Source: CAD feature listing. Evaluate the final solid. Frame: model axes, mm. Give positions to 0.01 mm unless a question says otherwise; leave off trailing zeros. Order: outer loops, then holes, each group sorted by start corner. A loop starts at its lowest first (then second) coordinate and runs counter-clockwise, first axis right, second up. Notation, with made-up numbers: M 23.25,73 L 80.25,73 A20 cw 80.25,112 Z; hole C -2.5,34.5 d5. An arc over 180 degrees is marked long. Answer as a JSON object with one key per item and string values. Group by question number.
1. Material intervals for L1, parallel to Y at x = 37, z = 0.25; L2, parallel to Y at x = 68, z = 0.8; L3, parallel to X at y = 65, z = 1.2 (3 decimals), sorted ascending. Write a range as [from, to].
2. Section query C-C (x = 57.15). Output: boundary loops of the cut face in (y, z), plus the area to 3 significant figures.
3. Section query A-A (x = 38). Output: boundary loops of the cut face in (y, z).
4. Section query D-D (y = 57). Output: boundary loops of the cut face in (x, z) (3 decimals).
5. Section query B-B (y = 68.35). Output: boundary loops of the cut face in (x, z) (3 decimals), plus the area to 3 significant figures.
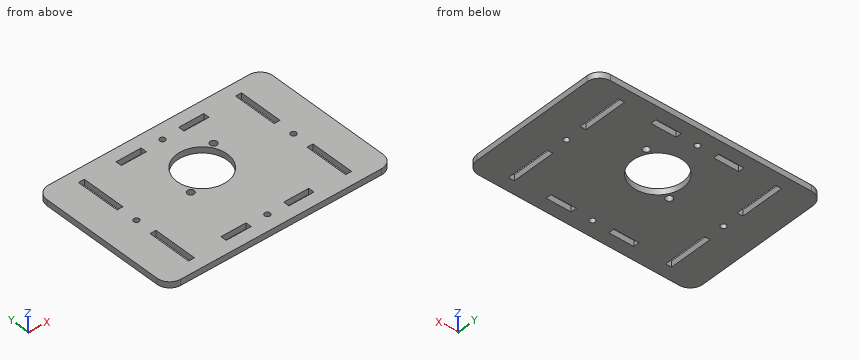
from build123d import *

# Parameters (mm, degrees)
BOSS_EXTRUDE1_DEPTH = 3
CUT_EXTRUDE1_REACH  = 139.404
SKETCH2_W           = 12.7
SKETCH2_H           = 3
SKETCH2_W_2         = 3
SKETCH2_H_2         = 22.225
CUT_EXTRUDE3_REACH  = 139.404
SKETCH4_R           = 1.7272
SKETCH4_R_2         = 12.70635
CUT_EXTRUDE4_REACH  = 139.404
SKETCH5_R           = 1.4097


with BuildPart() as part:
    # Sketch1 → Boss-Extrude1 (new body)
    with BuildSketch(Plane.XY):
        with BuildLine():
            Line((6.35, 0), (107.95, 0))
            ThreePointArc((107.95, 0), (112.440128061, 1.859871939), (114.3, 6.35))
            Line((114.3, 6.35), (114.3, 69.85))
            ThreePointArc((114.3, 69.85), (112.440128061, 74.340128061), (107.95, 76.2))
            Line((107.95, 76.2), (6.35, 76.2))
            ThreePointArc((6.35, 76.2), (1.859871939, 74.340128061), (0, 69.85))
            Line((0, 69.85), (0, 6.35))
            ThreePointArc((0, 6.35), (1.859871939, 1.859871939), (6.35, 0))
        make_face()
    extrude(amount=BOSS_EXTRUDE1_DEPTH)

    # Sketch2 → Cut-Extrude1 (cut, up to next)
    with BuildSketch(Plane(origin=(0, 0, 0), x_dir=(-1, 0, 0), z_dir=(0, 0, -1)), mode=Mode.PRIVATE) as cut_extrude1_sk1:
        with Locations((-73.025, 68.35)):
            Rectangle(SKETCH2_W, SKETCH2_H)
    cut_extrude1_tool1 = extrude(cut_extrude1_sk1.sketch, amount=-CUT_EXTRUDE1_REACH, mode=Mode.PRIVATE) & part.part
    # Sketch2 → Cut-Extrude1 (cut, up to next)
    with BuildSketch(Plane(origin=(0, 0, 0), x_dir=(-1, 0, 0), z_dir=(0, 0, -1)), mode=Mode.PRIVATE) as cut_extrude1_sk2:
        with Locations((-41.275, 68.35)):
            Rectangle(SKETCH2_W, SKETCH2_H)
    cut_extrude1_tool2 = extrude(cut_extrude1_sk2.sketch, amount=-CUT_EXTRUDE1_REACH, mode=Mode.PRIVATE) & part.part
    # Sketch2 → Cut-Extrude1 (cut, up to next)
    with BuildSketch(Plane(origin=(0, 0, 0), x_dir=(-1, 0, 0), z_dir=(0, 0, -1)), mode=Mode.PRIVATE) as cut_extrude1_sk3:
        with Locations((-17.375, 58.7375)):
            Rectangle(SKETCH2_W_2, SKETCH2_H_2)
    cut_extrude1_tool3 = extrude(cut_extrude1_sk3.sketch, amount=-CUT_EXTRUDE1_REACH, mode=Mode.PRIVATE) & part.part
    # Sketch2 → Cut-Extrude1 (cut, up to next)
    with BuildSketch(Plane(origin=(0, 0, 0), x_dir=(-1, 0, 0), z_dir=(0, 0, -1)), mode=Mode.PRIVATE) as cut_extrude1_sk4:
        with Locations((-17.375, 17.4625)):
            Rectangle(SKETCH2_W_2, SKETCH2_H_2)
    cut_extrude1_tool4 = extrude(cut_extrude1_sk4.sketch, amount=-CUT_EXTRUDE1_REACH, mode=Mode.PRIVATE) & part.part
    # Sketch2 → Cut-Extrude1 (cut, up to next)
    with BuildSketch(Plane(origin=(0, 0, 0), x_dir=(-1, 0, 0), z_dir=(0, 0, -1)), mode=Mode.PRIVATE) as cut_extrude1_sk5:
        with Locations((-41.275, 7.85)):
            Rectangle(SKETCH2_W, SKETCH2_H)
    cut_extrude1_tool5 = extrude(cut_extrude1_sk5.sketch, amount=-CUT_EXTRUDE1_REACH, mode=Mode.PRIVATE) & part.part
    # Sketch2 → Cut-Extrude1 (cut, up to next)
    with BuildSketch(Plane(origin=(0, 0, 0), x_dir=(-1, 0, 0), z_dir=(0, 0, -1)), mode=Mode.PRIVATE) as cut_extrude1_sk6:
        with Locations((-73.025, 7.85)):
            Rectangle(SKETCH2_W, SKETCH2_H)
    cut_extrude1_tool6 = extrude(cut_extrude1_sk6.sketch, amount=-CUT_EXTRUDE1_REACH, mode=Mode.PRIVATE) & part.part
    # Sketch2 → Cut-Extrude1 (cut, up to next)
    with BuildSketch(Plane(origin=(0, 0, 0), x_dir=(-1, 0, 0), z_dir=(0, 0, -1)), mode=Mode.PRIVATE) as cut_extrude1_sk7:
        with Locations((-96.925, 17.4625)):
            Rectangle(SKETCH2_W_2, SKETCH2_H_2)
    cut_extrude1_tool7 = extrude(cut_extrude1_sk7.sketch, amount=-CUT_EXTRUDE1_REACH, mode=Mode.PRIVATE) & part.part
    # Sketch2 → Cut-Extrude1 (cut, up to next)
    with BuildSketch(Plane(origin=(0, 0, 0), x_dir=(-1, 0, 0), z_dir=(0, 0, -1)), mode=Mode.PRIVATE) as cut_extrude1_sk8:
        with Locations((-96.925, 58.7375)):
            Rectangle(SKETCH2_W_2, SKETCH2_H_2)
    cut_extrude1_tool8 = extrude(cut_extrude1_sk8.sketch, amount=-CUT_EXTRUDE1_REACH, mode=Mode.PRIVATE) & part.part
    add(cut_extrude1_tool1.solids().sort_by_distance((73.025, 68.35, 0))[0], mode=Mode.SUBTRACT)
    add(cut_extrude1_tool2.solids().sort_by_distance((41.275, 68.35, 0))[0], mode=Mode.SUBTRACT)
    add(cut_extrude1_tool3.solids().sort_by_distance((17.375, 58.7375, 0))[0], mode=Mode.SUBTRACT)
    add(cut_extrude1_tool4.solids().sort_by_distance((17.375, 17.4625, 0))[0], mode=Mode.SUBTRACT)
    add(cut_extrude1_tool5.solids().sort_by_distance((41.275, 7.85, 0))[0], mode=Mode.SUBTRACT)
    add(cut_extrude1_tool6.solids().sort_by_distance((73.025, 7.85, 0))[0], mode=Mode.SUBTRACT)
    add(cut_extrude1_tool7.solids().sort_by_distance((96.925, 17.4625, 0))[0], mode=Mode.SUBTRACT)
    add(cut_extrude1_tool8.solids().sort_by_distance((96.925, 58.7375, 0))[0], mode=Mode.SUBTRACT)

    # Sketch4 → Cut-Extrude3 (cut, up to next)
    with BuildSketch(Plane.XY.offset(3), mode=Mode.PRIVATE) as cut_extrude3_sk1:
        with Locations((70.231, 53.822979832)):
            Circle(SKETCH4_R)
    cut_extrude3_tool1 = extrude(cut_extrude3_sk1.sketch, amount=-CUT_EXTRUDE3_REACH, mode=Mode.PRIVATE) & part.part
    # Sketch4 → Cut-Extrude3 (cut, up to next)
    with BuildSketch(Plane.XY.offset(3), mode=Mode.PRIVATE) as cut_extrude3_sk2:
        with Locations((44.069, 37.160579832)):
            Circle(SKETCH4_R)
    cut_extrude3_tool2 = extrude(cut_extrude3_sk2.sketch, amount=-CUT_EXTRUDE3_REACH, mode=Mode.PRIVATE) & part.part
    # Sketch4 → Cut-Extrude3 (cut, up to next)
    with BuildSketch(Plane.XY.offset(3), mode=Mode.PRIVATE) as cut_extrude3_sk3:
        with Locations((57.15, 45.491779832)):
            Circle(SKETCH4_R_2)
    cut_extrude3_tool3 = extrude(cut_extrude3_sk3.sketch, amount=-CUT_EXTRUDE3_REACH, mode=Mode.PRIVATE) & part.part
    add(cut_extrude3_tool1.solids().sort_by_distance((70.231, 53.82298, 3))[0], mode=Mode.SUBTRACT)
    add(cut_extrude3_tool2.solids().sort_by_distance((44.069, 37.16058, 3))[0], mode=Mode.SUBTRACT)
    add(cut_extrude3_tool3.solids().sort_by_distance((57.15, 45.49178, 3))[0], mode=Mode.SUBTRACT)

    # Sketch5 → Cut-Extrude4 (cut, up to next)
    with BuildSketch(Plane.XY.offset(3), mode=Mode.PRIVATE) as cut_extrude4_sk1:
        with Locations((57.15, 68.35)):
            Circle(SKETCH5_R)
    cut_extrude4_tool1 = extrude(cut_extrude4_sk1.sketch, amount=-CUT_EXTRUDE4_REACH, mode=Mode.PRIVATE) & part.part
    # Sketch5 → Cut-Extrude4 (cut, up to next)
    with BuildSketch(Plane.XY.offset(3), mode=Mode.PRIVATE) as cut_extrude4_sk2:
        with Locations((96.925, 38.1)):
            Circle(SKETCH5_R)
    cut_extrude4_tool2 = extrude(cut_extrude4_sk2.sketch, amount=-CUT_EXTRUDE4_REACH, mode=Mode.PRIVATE) & part.part
    # Sketch5 → Cut-Extrude4 (cut, up to next)
    with BuildSketch(Plane.XY.offset(3), mode=Mode.PRIVATE) as cut_extrude4_sk3:
        with Locations((57.15, 7.85)):
            Circle(SKETCH5_R)
    cut_extrude4_tool3 = extrude(cut_extrude4_sk3.sketch, amount=-CUT_EXTRUDE4_REACH, mode=Mode.PRIVATE) & part.part
    # Sketch5 → Cut-Extrude4 (cut, up to next)
    with BuildSketch(Plane.XY.offset(3), mode=Mode.PRIVATE) as cut_extrude4_sk4:
        with Locations((17.375, 38.1)):
            Circle(SKETCH5_R)
    cut_extrude4_tool4 = extrude(cut_extrude4_sk4.sketch, amount=-CUT_EXTRUDE4_REACH, mode=Mode.PRIVATE) & part.part
    add(cut_extrude4_tool1.solids().sort_by_distance((57.15, 68.35, 3))[0], mode=Mode.SUBTRACT)
    add(cut_extrude4_tool2.solids().sort_by_distance((96.925, 38.1, 3))[0], mode=Mode.SUBTRACT)
    add(cut_extrude4_tool3.solids().sort_by_distance((57.15, 7.85, 3))[0], mode=Mode.SUBTRACT)
    add(cut_extrude4_tool4.solids().sort_by_distance((17.375, 38.1, 3))[0], mode=Mode.SUBTRACT)


solid = part.part
Answer sheet:
{
 "1": {"L1": "[0, 6.35], [9.35, 66.85], [69.85, 76.2]", "L2": "[0, 6.35], [9.35, 38.88], [52.1, 66.85], [69.85, 76.2]", "L3": "[0, 15.875], [18.875, 95.425], [98.425, 114.3]"},
 "2": {"outline": "M 0,0 L 6.44,0 L 6.44,3 L 0,3 Z; M 9.26,0 L 32.79,0 L 32.79,3 L 9.26,3 Z; M 58.2,0 L 66.94,0 L 66.94,3 L 58.2,3 Z; M 69.76,0 L 76.2,0 L 76.2,3 L 69.76,3 Z", "area": "135 mm^2"},
 "3": {"outline": "M 0,0 L 6.35,0 L 6.35,3 L 0,3 Z; M 9.35,0 L 66.85,0 L 66.85,3 L 9.35,3 Z; M 69.85,0 L 76.2,0 L 76.2,3 L 69.85,3 Z"},
 "4": {"outline": "M 0,0 L 15.875,0 L 15.875,3 L 0,3 Z; M 18.875,0 L 51.764,0 L 51.764,3 L 18.875,3 Z; M 62.536,0 L 95.425,0 L 95.425,3 L 62.536,3 Z; M 98.425,0 L 114.3,0 L 114.3,3 L 98.425,3 Z"},
 "5": {"outline": "M 0,0 L 15.875,0 L 15.875,3 L 0,3 Z; M 18.875,0 L 34.925,0 L 34.925,3 L 18.875,3 Z; M 47.625,0 L 55.74,0 L 55.74,3 L 47.625,3 Z; M 58.56,0 L 66.675,0 L 66.675,3 L 58.56,3 Z; M 79.375,0 L 95.425,0 L 95.425,3 L 79.375,3 Z; M 98.425,0 L 114.3,0 L 114.3,3 L 98.425,3 Z", "area": "240 mm^2"}
}
